Autodesk Inventor part; units mm, degrees
ref_plane "Pracovní rovina1" through (0, 0, -7.5) normal (0, 0, -1) x (-1, 0, 0)
ref_plane "YZ Plane" through (0, 0, 0) normal (1, 0, 0) x (0, 1, 0)
ref_plane "XZ Plane" through (0, 0, 0) normal (0, 1, 0) x (-1, 0, 0)
sketch "Náčrt1" plane through (0, 0, 0) normal (0, 1, 0) x (-1, 0, 0)
  line L0 (0, 0) -> (0, -15)
  line L1 (0, -15) -> (18, -15)
  line L2 (18, -15) -> (18, 0)
  line L3 (18, 0) -> (0, 0)
  dimension "d0" = 15
  dimension "d1" = 18
extrude "Vysunutí1" add sketch "Náčrt1" along normal blind 8
sketch "Náčrt2" plane through (0, 0, 0) normal (1, 0, 0) x (0, 0, -1)
  line L0 (0, 0) -> (15, 0)
  line L1 (15, 0) -> (15, 8)
  line L2 (0, 8) -> (15, 8)
  line L3 (0, 0) -> (0, 8)
  circle A0 centre (12.5, 4) radius 1.4
  line L4 (15, 8) -> (0, 8)
  line L5 (7.5, 8) -> (7.5, 0) construction
  circle A1 centre (2.5, 4) radius 1.4
  point P0 (15, 4)
  dimension "d4" = 10
  dimension "d7" = 2.8
extrude "Vysunutí2" cut sketch "Náčrt2" against normal blind 10 contours A0 | A1
sketch "Náčrt3" plane through (-18, 0, -15) normal (-1, 0, 0) x (0, 0, 1)
  line L0 (0, 0) -> (15, 0)
  line L1 (15, 0) -> (15, 8)
  line L2 (0, 8) -> (15, 8)
  line L3 (0, 0) -> (0, 8)
  circle A0 centre (7.5, 4) radius 1.1
  point P0 (15, 0)
  dimension "d8" = 2.2
extrude "Vysunutí3" cut sketch "Náčrt3" against normal through all contours A0
ref_plane "Pracovní rovina1" through (0, 0, -7.5) normal (0, 0, -1) x (-1, 0, 0)
sketch "Náčrt4" plane through (0, 0, -7.5) normal (0, 0, -1) x (-1, 0, 0)
  line L0 (0, 0) -> (18, 0)
  line L1 (18, 0) -> (18, 8)
  line L2 (0, 8) -> (18, 8)
  line L3 (0, 0) -> (0, 8)
  line L4 (1, 8) -> (8, 1)
  line L5 (8, 1) -> (15, 8)
  point P0 (0, 0)
  dimension "d11" = 90
  dimension "d12" = 7
  dimension "d15" = 8
extrude "Vysunutí4" cut sketch "Náčrt4" along normal mid plane 6 contours L2 L5 L4
properties part number "uchyceni_pruziny"
Check sheet for the modelled part. Datum: model origin and axes. Units: mm. A direction names the side the tool comes from. Give positions to 0.01 mm unless a question says otherwise; leave off trailing zeros. Order: outer loops, then holes, each group sorted by start corner. A loop starts at its lowest first (then second) coordinate and runs counter-clockwise, first axis right, second up. Notation, with made-up numbers: (83, 76.25) -> (92, 76.25) arc R14 cw to (92, 85.25) -> close; hole circle Ø6 at (54, 28.25). An arc over 180 degrees is marked (long way). Use CSV: the item, a comma, the result in double quotes. Start each with the question number.
1) Set-up check for faces 5 (the face through (-8, 5, -4.5)), 6 (the face through (0, 4, -6)), 7 (the face through (-4.93, 2.76, -3.15)): record each of +Z, -Z, +X, -X, +Y, -Y from which the full face is reachable in a straight line by a thin tool's end or side.
2) Mould release check, pull along X, two halves, no side actions. Record for faces 1 (the face through (-12.2, 5.2, -8.1)), 2 (the face through (-8, 5, -10.5)), 3 (the face through (-4.93, 4.06, -11.1)), 4 (the face through (-18, 4, -9)): released by +X, released by -X, zero draft, split by the parting line, or undercut.
3) Sectioned sample at A-A, the plane z = -7.5. Record the boundary of the cut face in (x, y), plus the area to 3 significant figures.
4) Sectioned sample at D-D, the plane x = -14.75. Record the boundary of the cut face in (y, z), plus the area to 3 significant figures.
5) Go/stop test with a flat-tipped pin: P1, Ø1.8, axis at y = 4, z = -7.5, coming from the +X side. Record where the tip stops, or that it passes through.
6) Material ranges on line 1 (Z direction, x = -11, y = 4.25); line 2 (Z direction, x = -11.75, y = 4); line 3 (Y direction, x = -4, z = -1.5), recorded low to high. Write a range as from..to.
7) Sectioned sample at B-B, the plane x = -7.5. Record the boundary of the cut face in (y, z).
8) Sectioned sample at C-C, the plane y = 1.5. Record the boundary of the cut face in (x, z).
Recorded:
1,face 5,"+Y"
1,face 6,"+Z, -Z, +X, +Y, -Y"
1,face 7,"+X"
2,face 1,"undercut"
2,face 2,"undercut"
2,face 3,"zero draft"
2,face 4,"released by -X"
3,outline,"(-18, 0) -> (0, 0) -> (0, 2.9) -> (-6.1, 2.9) -> (-8, 1) -> (-9.9, 2.9) -> (-18, 2.9) -> close; (-18, 5.1) -> (-12.1, 5.1) -> (-15, 8) -> (-18, 8) -> close; (-3.9, 5.1) -> (0, 5.1) -> (0, 8) -> (-1, 8) -> close"
3,area,"68.6 mm2"
4,outline,"(0, -15) -> (8, -15) -> (8, -10.5) -> (7.75, -10.5) -> (7.75, -4.5) -> (8, -4.5) -> (8, 0) -> (0, 0) -> close; hole circle Ø2.2 at (4, -7.5)"
4,area,"115 mm2"
5,P1,"through"
6,line 1,"-15..-10.5, -4.5..0"
6,line 2,"-15..-8.6, -6.4..0"
6,line 3,"0..3.02, 4.98..8"
7,outline,"(0, -15) -> (8, -15) -> (8, -10.5) -> (1.5, -10.5) -> (1.5, -4.5) -> (8, -4.5) -> (8, 0) -> (0, 0) -> close; hole circle Ø2.8 at (4, -12.5); hole circle Ø2.8 at (4, -2.5)"
8,outline,"(-18, -15) -> (0, -15) -> (0, 0) -> (-18, 0) -> close; hole (-8.5, -10.5) -> (-7.5, -10.5) -> (-7.5, -4.5) -> (-8.5, -4.5) -> close"
